Geometry check sheet. Reference: the model listing, model coordinates, mm. Coordinates: 2 decimals unless noted, no trailing zeros.
from build123d import *

# Parameters (mm, degrees)
BOSS_EXTRUDE2_DEPTH     = 3.25
CUT_EXTRUDE4_DEPTH      = 11.447288324
CUT_EXTRUDE4_DEPTH_BACK = 11.447288324
SKETCH16_R              = 4
SKETCH7_OUTSIDE_W       = 63.752
SKETCH7_OUTSIDE_H       = 65.764
SKETCH7_OUTSIDE_R       = 6.5
CUT_EXTRUDE5_DEPTH      = 12.867322079
CUT_EXTRUDE5_DRAFT      = -60
MIRROR4_COPY_1_SKETCH_W = 63.752
MIRROR4_COPY_1_SKETCH_H = 65.764
MIRROR4_COPY_1_SKETCH_R = 6.5
MIRROR4_COPY_1_DEPTH    = 12.867322079
MIRROR4_COPY_1_DRAFT    = -60
FILLET2_R               = 0.325


with BuildPart() as part:
    # Sketch15 → Boss-Extrude2 (new, symmetric)
    with BuildSketch(Plane.XY):
        Polygon((0, 7.505553499), (-6.5, 3.75277675), (-6.5, -3.75277675), (0, -7.505553499), (6.5, -3.75277675), (6.5, 3.75277675), align=None)
    extrude(amount=BOSS_EXTRUDE2_DEPTH, both=True)

    # Sketch16 → Cut-Extrude4 (cut, two sides: drawn at the far end of the back side and taken through both)
    with BuildSketch(Plane.XY.offset(-CUT_EXTRUDE4_DEPTH_BACK)):
        Circle(SKETCH16_R)
    extrude(amount=CUT_EXTRUDE4_DEPTH + CUT_EXTRUDE4_DEPTH_BACK, mode=Mode.SUBTRACT)


with BuildPart() as cut_extrude5_tool:
    # Sketch7 outside → Cut-Extrude5 (with draft: the straight prism first)
    with BuildSketch(Plane.XY.offset(3.25)):
        Rectangle(SKETCH7_OUTSIDE_W, SKETCH7_OUTSIDE_H)
        Circle(SKETCH7_OUTSIDE_R, mode=Mode.SUBTRACT)
    extrude(amount=-CUT_EXTRUDE5_DEPTH)
    # Cut-Extrude5: the draft: its side faces are tilted about the plane it starts from
    cut_extrude5_sides = [cut_extrude5_tool.faces().sort_by_distance(p)[0] for p in [
        (0, -32.882, -3.18366104),
        (31.876, 0, -3.18366104),
        (0, 32.882, -3.18366104),
        (-31.876, 0, -3.18366104),
        (-6.5, 0, -3.18366104),
    ]]
    draft(cut_extrude5_sides, Plane.XY.offset(3.25), CUT_EXTRUDE5_DRAFT)


with BuildPart() as part_1:
    add(part.part)

    # Cut-Extrude5: cut by cut_extrude5_tool
    add(cut_extrude5_tool.part, mode=Mode.SUBTRACT)


with BuildPart() as mirror4_copy_1_tool:
    # Mirror4 copy 1 sketch → Mirror4 copy 1 (with draft: the straight prism first)
    with BuildSketch(Plane(origin=(0, 0, -3.25), x_dir=(1, 0, 0), z_dir=(0, 0, -1))):
        Rectangle(MIRROR4_COPY_1_SKETCH_W, MIRROR4_COPY_1_SKETCH_H)
        Circle(MIRROR4_COPY_1_SKETCH_R, mode=Mode.SUBTRACT)
    extrude(amount=-MIRROR4_COPY_1_DEPTH)
    # Mirror4 copy 1: the draft: its side faces are tilted about the plane it starts from
    mirror4_copy_1_sides = [mirror4_copy_1_tool.faces().sort_by_distance(p)[0] for p in [
        (0, -32.882, 3.18366104),
        (31.876, 0, 3.18366104),
        (0, 32.882, 3.18366104),
        (-31.876, 0, 3.18366104),
        (-6.5, 0, 3.18366104),
    ]]
    draft(mirror4_copy_1_sides, Plane(origin=(0, 0, -3.25), x_dir=(1, 0, 0), z_dir=(0, 0, -1)), MIRROR4_COPY_1_DRAFT)


with BuildPart() as part_2:
    add(part_1.part)

    # Mirror4 copy 1: cut by mirror4_copy_1_tool
    add(mirror4_copy_1_tool.part, mode=Mode.SUBTRACT)

    # Fillet2
    fillet2_edges = [part_2.edges().sort_by_distance(p)[0] for p in [
        (-6.5, 3.75277675, 0),
        (-6.5, -3.75277675, 0),
        (0, -7.505553499, 0),
        (6.5, -3.75277675, 0),
        (6.5, 3.75277675, 0),
        (0, 7.505553499, 0),
    ]]
    fillet(fillet2_edges, radius=FILLET2_R)


solid = part_2.part
1) Depth check by flat-ended pin: pin 1 (3 mm diameter, centred on x = 1.5, y = 0.5, fed in from -Z); pin 2 (1 mm diameter, centred on x = 2, z = 0, fed in from -Y). Enter the tip coordinate at first touch or a pass-through.
Data:
pin 1: passes through
pin 2: stops at y = -6.64
2) Material ranges on probe 1 along Y at (x, z) = (0, -2); probe 2 along X at (y, z) = (0, -1.5); probe 3 along Y at (x, z) = (-3.5, 2.5), recorded low to high.
Data:
probe 1: y = -7.46 to -4, 4 to 7.46
probe 2: x = -6.5 to -4, 4 to 6.5
probe 3: y = -5.48 to -1.94, 1.94 to 5.48
3) Mould release check, pull along X, two halves, no side actions. Record for faces 1 (the conical face through (-5.83, -3.35, 3.12)), 2 (the flat face through (3.3, 5.6, 0)), 3 (the cylindrical face through (-0.867, -3.905, -0.046)): +X half, -X half, draft (parallel to the pull), parting line (faces both ways), or undercut.
Data:
face 1: -X half
face 2: +X half
face 3: undercut
